Source: CAD feature listing. Evaluate the final solid. Frame: model axes, mm. A direction names the side the tool comes from. Give positions to 0.01 mm unless a question says otherwise; leave off trailing zeros. Order: outer loops, then holes, each group sorted by start corner. A loop starts at its lowest first (then second) coordinate and runs counter-clockwise, first axis right, second up. Notation, with made-up numbers: M -11.75,55 L 3.25,55 A8 ccw 3.25,61 Z; hole C 31,-1 d1. An arc over 180 degrees is marked long. Answer in a Markdown table with one row per item. Add a question column.
(1) Material intervals for line 1 along Z through (x, y) = (-165.5, 106); line 2 along Y through (x, z) = (-154, 26); line 3 along Y through (x, z) = (-131, 31), sorted ascending.
(2) Section query C-C, the plane y = 128.5. Return loops of the section in (x, z).
(3) Section query D-D, the plane z = 20. Return loops of the section in (x, y).
(4) Section query A-A, the plane y = 72.5. Return loops of the section in (x, z), plus the area to 3 significant figures.
(5) Pin query (flat end, axial travel): P1, Ø3.5, axis at x = -165, z = 31, coming from the +Y side; P2, Ø8, axis at x = -103.5, z = 19.5, coming from the +Y side; P3, Ø8, axis at x = -108.5, z = 16.5, coming from the -Y side; P4, Ø10, axis at y = 129, z = 21.5, coming from the -X side. Return the tip coordinate at first contact, or that it passes through.
(6) Section query B-B, the plane x = -169.5. Return loops of the section in (y, z), plus the area to 3 significant figures.
(7) Mould query, pull axis Z, two halves, no side actions, for faces 1 (the face through (-128, 76.67, 16)), 2 (the face through (-182.955, 113.12, 31.479)), 3 (the face through (-135, 95, 0)). Classes: pulls with the +Z half, pulls with the -Z half, needs draft (parallel to the pull), parting line crosses it, or undercut.
(8) Set-up query: faces 4 (the face through (-124, 103, 30)), 5 (the face through (-178.222, 79, 14)), 6 (the face through (-108.08, 128.01, 1.48)). Return all of +Z, -Z, +X, -X, +Y, -Y with unobstructed straight access to the full face (end or side cutting, diameter ignored); none if empty.
from build123d import *

# Parameters (mm, degrees)
F0_R      = 5
F1_DEPTH  = 33
F5_W      = 100
F5_H      = 3
F6_DEPTH  = 28
F7_W      = 100
F7_H      = 3
F8_DEPTH  = 10
F7_H_2    = 33
F13_DEPTH = 116.001
F14_W     = 100
F14_H     = 3
F15_DEPTH = 10
F18_DEPTH = 33.001
F21_DEPTH = 33.001
F24_DEPTH = 33.001
F25_SIZE  = 2


with BuildPart() as f1:
    # F0 (on Top) → F1 (new body)
    with BuildSketch(Plane.XY):
        with BuildLine():
            Line((21.777506699, 52.6698508731), (21.777506699, 56.6698508731))
            Line((21.777506699, 56.6698508731), (-78.222493301, 56.6698508731))
            Line((-78.222493301, 56.6698508731), (-78.222493301, 16.6698508731))
            Line((-78.222493301, 16.6698508731), (-58.222493301, -5.6908289019))
            Line((-58.222493301, -5.6908289019), (-38.222493301, 16.6698508731))
            Line((-38.222493301, 16.6698508731), (-18.222493301, -5.6908289019))
            Line((-18.222493301, -5.6908289019), (1.777506699, 16.6698508731))
            Line((1.777506699, 16.6698508731), (21.777506699, 16.6698508731))
            Line((21.777506699, 16.6698508731), (31.377506699, 23.8698508731))
            ThreePointArc((31.377506699, 23.8698508731), (36.9564394679, 41.7294951294), (21.777506699, 52.6698508731))
        make_face()
        with Locations((21.777506699, 36.6698508731)):
            Circle(F0_R, mode=Mode.SUBTRACT)
    extrude(amount=F1_DEPTH)


with BuildPart() as f2_1:
    # F2: copy of F1
    add(f1.part.moved(Location((0, 0, 28))))


with BuildPart() as f4_1:
    # F4: copy of F1
    add(f1.part.moved(Location((0, 0, 34))))


with BuildPart() as f6:
    # F5 (on face) → F6 (new body)
    with BuildSketch(Plane.XY.offset(33)):
        with Locations((-28.222493301, 55.1698508731)):
            Rectangle(F5_W, F5_H)
    extrude(amount=F6_DEPTH)


with BuildPart() as f8:
    # F7 (on face) → F8 (new body)
    with BuildSketch(Plane(origin=(0, 56.6698508731, 0), x_dir=(-1, 0, 0), z_dir=(0, 1, 0))):
        with Locations((28.222493301, 62.5)):
            Rectangle(F7_W, F7_H)
    extrude(amount=F8_DEPTH)


with BuildPart() as f8b:
    # F7 (on face) → F8, piece 2 (new body)
    with BuildSketch(Plane(origin=(0, 56.6698508731, 0), x_dir=(-1, 0, 0), z_dir=(0, 1, 0))):
        with Locations((28.222493301, 16.5)):
            Rectangle(F7_W, F7_H_2)
    extrude(amount=F8_DEPTH)


with BuildPart() as f1_1:
    add(f1.part)

    # F12 (on face) → F13 (cut, through all)
    with BuildSketch(Plane(origin=(-78.222493301, 0, 0), x_dir=(0, -1, 0), z_dir=(-1, 0, 0))):
        Polygon((15.5293103307, 30), (-53.6698508731, 30), (-53.6698508731, 3), (13.7041052803, 3), align=None)
    extrude(amount=-F13_DEPTH, mode=Mode.SUBTRACT)

    # F14 (on face) → F15 (join)
    with BuildSketch(Plane(origin=(0, 56.6698508731, 0), x_dir=(-1, 0, 0), z_dir=(0, 1, 0))):
        with Locations((28.222493301, 1.5)):
            Rectangle(F14_W, F14_H)
        with Locations((28.222493301, 31.5)):
            Rectangle(F14_W, F14_H)
    extrude(amount=F15_DEPTH)

    # F16: F1 across face


with BuildPart() as f1_2:
    add(f1_1.part)
    add(f1_1.part.mirror(Plane(origin=(-78.222493301, 44.5399296132, 16.5), x_dir=(0, -1, 0), z_dir=(-1, 0, 0))))

    # F17 (on face) → F18 (cut, through all)
    with BuildSketch(Plane.XY.offset(33)):
        Polygon((-78.222493301, 86.7001339793), (-78.222493301, 16.6698508731), (-78.222493301, -27.7220606804), (68.2113543153, -27.7220606804), (68.2113543153, 86.7001339793), align=None)
    extrude(amount=-F18_DEPTH, mode=Mode.SUBTRACT)

    # F19: F1 across face


with BuildPart() as f1_3:
    add(f1_2.part)
    add(f1_2.part.mirror(Plane(origin=(-78.222493301, 44.5399296132, 16.5), x_dir=(0, 1, 0), z_dir=(1, 0, 0))))

    # F20 (on face) → F21 (cut, through all)
    with BuildSketch(Plane.XY.offset(33)):
        Polygon((54.2253777385, 66.6698508731), (-78.222493301, 66.6698508731), (-78.222493301, -28.4001789987), (54.2253777385, -31.8515859544), align=None)
    extrude(amount=-F21_DEPTH, mode=Mode.SUBTRACT)

    # F22: F1 across face


with BuildPart() as f1_4:
    add(f1_3.part)
    add(f1_3.part.mirror(Plane(origin=(-128.222493301, 66.6698508731, 31.5), x_dir=(-1, 0, 0), z_dir=(0, 1, 0))))

    # F23 (on face) → F24 (cut, through all)
    with BuildSketch(Plane.XY.offset(33)):
        Polygon((-78.222493301, -18.2117372751), (-78.222493301, 66.6698508731), (-239.6576553583, 66.6698508731), (-202.1560966969, -18.2117372751), align=None)
    extrude(amount=-F24_DEPTH, mode=Mode.SUBTRACT)

    # F25
    f25_edges = [f1_4.edges().sort_by_distance(p)[0] for p in [
        (-178.222493, 76.669851, 16.5),
        (-78.222493, 76.669851, 16.5),
    ]]
    chamfer(f25_edges, length=F25_SIZE)


solid = f1_4.part
Values follow:
| question | item | result |
|---|---|---|
| 1 | line 1 | z = 0 to 3, 30 to 33 |
| 1 | line 2 | y = 76.67 to 79.67 |
| 1 | line 3 | y = 66.67 to 130.96 |
| 2 | outline | M -147.64,0 L -128.8,0 L -128.8,3 L -147.64,3 Z; M -147.64,30 L -128.8,30 L -128.8,33 L -147.64,33 Z; M -107.64,0 L -88.8,0 L -88.8,3 L -107.64,3 Z; M -107.64,30 L -88.8,30 L -88.8,33 L -107.64,33 Z |
| 3 | outline | M -178.22,78.67 L -176.22,76.67 L -80.22,76.67 L -78.22,78.67 L -78.22,79.67 L -178.22,79.67 Z |
| 4 | outline | M -178.22,0 L -78.22,0 L -78.22,3 L -178.22,3 Z; M -178.22,30 L -78.22,30 L -78.22,33 L -178.22,33 Z |
| 4 | area | 600 mm² |
| 5 | P1 | stops at y = 116.67 |
| 5 | P2 | stops at y = 79.67 |
| 5 | P3 | stops at y = 76.67 |
| 5 | P4 | passes through |
| 6 | outline | M 66.67,0 L 116.67,0 L 116.67,3 L 79.67,3 L 79.67,30 L 116.67,30 L 116.67,33 L 66.67,33 L 66.67,30 L 76.67,30 L 76.67,3 L 66.67,3 Z |
| 6 | area | 381 mm² |
| 7 | face 1 | undercut |
| 7 | face 2 | needs draft |
| 7 | face 3 | pulls with the -Z half |
| 8 | face 4 | +X, -X, +Y |
| 8 | face 5 | +Z, -Z, -X, -Y |
| 8 | face 6 | +Z, -Z, +Y |
